The listing builds one solid part. Answer for the finished solid, in the listing's coordinates (mm). A direction names the side the tool comes from. Coordinates: 2 decimals unless noted, no trailing zeros. Write each loop counter-clockwise with the first axis right and the second up, starting at its lowest first coordinate (ties: lowest second). Pieces come first, ordered by that corner, then holes.
(1) Which of the six approach directions +Z, -Z, +X, -X, +Y, -Y give full straight-line access (tool end or side, diameter ignored) to faces 3 (the cylindrical face through (-0.4, 64.3, 7.5)), 4 (the flat face through (67, 25, 5)), 5 (the flat face through (-55, 46, 5)), 6 (the flat face through (-12, -71, 5))?
(2) The part is cut by section B-B on y = 0. Determine the outline of the cut face in (x, z), plus the area to 3 significant figures.
(3) Straight lines are drawn through the part: line 1 (Y direction, x = 0, z = 8.25); line 2 (Y direction, x = 22, z = 8); line 3 (X direction, y = 54, z = 1.25). For each, find the intervals that lie inside material, in ascending order.
(4) Given P1, Ø5.5, axis at x = -56.69, y = 47.57, coming from the -Z side; P2, Ø3, axis at y = -20.5, z = 8.5, coming from the -X side; P3, Ø5, axis at y = -4, z = 6.5, coming from the +X side; P4, Ø2, axis at x = -12.85, y = -72.88, coming from the +Z side, each flat-ended and moving along its own axis, determine where each tip first touches the part or whether it passes through.
(5) The part is cut by section A-A on x = 0. Determine the outline of the cut face in (y, z), plus the area to 4 significant figures.
(6) The part is cut by section C-C on x = -17.5. Determine the outline of the cut face in (y, z), plus the area to 3 significant figures.
(7) For a pull along Y with two mould halves and no side action, classify faces 1 (the cylindrical face through (-59.48, 49.68, 7.46)), 2 (the flat face through (56, 31, 0)) as +Y half, -Y half, draft (parallel to the pull), parting line (faces both ways), or undercut.
from build123d import *

# Parameters (mm, degrees)
SCHIZZO1_R                   = 70
SCHIZZO1_R_2                 = 62.5
ESTRUSIONE_ESTRUSIONE1_DEPTH = 10
ESTRUSIONE_ESTRUSIONE3_START = -5
ESTRUSIONE_ESTRUSIONE3_DEPTH = 5
FORO_PER_VITE_M3_2_D         = 3.4
RIPETIZIONECIRCOLARE3_COUNT  = 3
SCHIZZO14_R                  = 62.5
TAGLIO_ESTRUSIONE1_DEPTH     = 30
RIPETIZIONECIRCOLARE4_COUNT  = 3


with BuildPart() as part:
    # Schizzo1 → Estrusione-Estrusione1 (new body)
    with BuildSketch(Plane.XY):
        Circle(SCHIZZO1_R)
        Circle(SCHIZZO1_R_2, mode=Mode.SUBTRACT)
    extrude(amount=ESTRUSIONE_ESTRUSIONE1_DEPTH)

    # Schizzo5 → Estrusione-Estrusione3 (add)
    with BuildSketch(Plane(origin=(0, 0, 0), x_dir=(-1, 0, 0), z_dir=(0, 0, -1)).offset(ESTRUSIONE_ESTRUSIONE3_START)):
        with BuildLine():
            ThreePointArc((4.710151164, -69.841352192), (13.457733769, -76.322600858), (19.461054995, -67.240369857))
            ThreePointArc((19.461054995, -67.240369857), (12.155372437, -68.936542711), (4.710151164, -69.841352192))
        make_face()
    estrusione_estrusione3 = extrude(amount=-ESTRUSIONE_ESTRUSIONE3_DEPTH)

    # Foro per Vite M3-2 (through all)
    with Locations(Plane(origin=(0, 0, 5), x_dir=(-1, 0, 0), z_dir=(0, 0, -1))):
        with Locations((12.849965147, -72.875773723)):
            foro_per_vite_m3_2 = Hole(FORO_PER_VITE_M3_2_D / 2)

    # RipetizioneCircolare3: Estrusione-Estrusione3, Foro per Vite M3-2 ×3 about axis
    ripetizionecircolare3_axis = Axis((0, 0, 0), (0, 0, 1))
    add([estrusione_estrusione3.rotate(ripetizionecircolare3_axis, i * 360 / RIPETIZIONECIRCOLARE3_COUNT) for i in range(1, RIPETIZIONECIRCOLARE3_COUNT)])
    add([foro_per_vite_m3_2.rotate(ripetizionecircolare3_axis, i * 360 / RIPETIZIONECIRCOLARE3_COUNT) for i in range(1, RIPETIZIONECIRCOLARE3_COUNT)], mode=Mode.SUBTRACT)

    # Schizzo14 → Taglio-Estrusione1 (cut)
    with BuildSketch(Plane(origin=(-60.621778265, -35, 0), x_dir=(0, 0, -1), z_dir=(-0.8660254037844398, -0.499999999999998, 0))):
        with Locations((55, 0)):
            Circle(SCHIZZO14_R)
    taglio_estrusione1 = extrude(amount=-TAGLIO_ESTRUSIONE1_DEPTH, mode=Mode.SUBTRACT)

    # RipetizioneCircolare4: Taglio-Estrusione1 ×3 about axis
    ripetizionecircolare4_axis = Axis((0, 0, 10), (0, 0, -1))
    for i in range(1, RIPETIZIONECIRCOLARE4_COUNT):
        add(taglio_estrusione1.rotate(ripetizionecircolare4_axis, i * 360 / RIPETIZIONECIRCOLARE4_COUNT), mode=Mode.SUBTRACT)


solid = part.part
Model answer:
1. face 3: -Z, +Y
1. face 4: -Z, +X, +Y
1. face 5: -Z, -X, +Y
1. face 6: -Z, -X, -Y
2. outline: (-70, 0) - (-62.5, 0) - (-62.5, 10) - (-70, 10) - close; (62.5, 0) - (70, 0) - (70, 10) - (62.5, 10) - close
2. area: 150 mm2
3. line 1: y = -70 to -62.5, 62.5 to 70
3. line 2: y = -66.45 to -58.5, 58.5 to 66.45
3. line 3: x = -44.54 to -31.47, 31.47 to 44.54
4. P1: stops at z = 5
4. P2: stops at x = -67.37
4. P3: stops at x = 69.98
4. P4: passes through
5. outline: (-70, 0) - (-62.5, 0) - (-62.5, 10) - (-70, 10) - close; (62.5, 7.5) - (70, 7.5) - (70, 10) - (62.5, 10) - close
5. area: 93.75 mm2
6. outline: (-74.2, 5) - (-67.78, 5) - (-67.78, 0) - (-60, 0) - (-60, 10) - (-74.2, 10) - close; (60, 5) - (67.78, 5) - (67.78, 10) - (60, 10) - close
6. area: 149 mm2
7. face 1: undercut
7. face 2: draft
